```python
from build123d import *

# Parameters (mm, degrees)
SKETCH1_W           = 2500
SKETCH1_H           = 700
SKETCH1_W_2         = 2440
SKETCH1_H_2         = 640
BOSS_EXTRUDE1_DEPTH = 1500
SKETCH2_W           = 2440
SKETCH2_H           = 1440
CUT_EXTRUDE1_DEPTH  = 1500
SKETCH3_W           = 1440
SKETCH3_H           = 640
CUT_EXTRUDE2_DEPTH  = 3595
SKETCH5_W           = 15
SKETCH5_H           = 30
BOSS_EXTRUDE3_DEPTH = 640
BOSS_EXTRUDE4_REACH = 2472
SKETCH7_W           = 30
SKETCH7_H           = 30
SKETCH8_W           = 30
SKETCH8_H           = 30
BOSS_EXTRUDE5_DEPTH = 640


with BuildPart() as part:
    # Sketch1 → Boss-Extrude1 (new body)
    with BuildSketch(Plane.XY):
        with Locations((1250, 350)):
            Rectangle(SKETCH1_W, SKETCH1_H)
        with Locations((1250, 350)):
            Rectangle(SKETCH1_W_2, SKETCH1_H_2, mode=Mode.SUBTRACT)
    extrude(amount=BOSS_EXTRUDE1_DEPTH)

    # Sketch2 → Cut-Extrude1 (cut)
    with BuildSketch(Plane(origin=(0, 700, 0), x_dir=(1, 0, 0), z_dir=(0, 1, 0))):
        with Locations((1250, -750)):
            Rectangle(SKETCH2_W, SKETCH2_H)
    extrude(amount=-CUT_EXTRUDE1_DEPTH, mode=Mode.SUBTRACT)

    # Sketch3 → Cut-Extrude2 (cut)
    with BuildSketch(Plane(origin=(2500, 0, 0), x_dir=(0, 0, -1), z_dir=(1, 0, 0))):
        with Locations((-750, 350)):
            Rectangle(SKETCH3_W, SKETCH3_H)
    extrude(amount=-CUT_EXTRUDE2_DEPTH, mode=Mode.SUBTRACT)

    # Sketch5 → Boss-Extrude3 (add)
    with BuildSketch(Plane(origin=(0, 30, 0), x_dir=(1, 0, 0), z_dir=(0, 1, 0))):
        with Locations((632.5, -15)):
            Rectangle(SKETCH5_W, SKETCH5_H)
        with Locations((647.5, -15)):
            Rectangle(SKETCH5_W, SKETCH5_H)
        with Locations((1242.5, -15)):
            Rectangle(SKETCH5_W, SKETCH5_H)
        with Locations((1257.5, -15)):
            Rectangle(SKETCH5_W, SKETCH5_H)
        Polygon((1860, 0), (1845, 0), (1845, -30), (1860, -30), (1875, -30), (1875, 0), align=None)
        with Locations((1852.5, -1485)):
            Rectangle(SKETCH5_W, SKETCH5_H)
        with Locations((1867.5, -1485)):
            Rectangle(SKETCH5_W, SKETCH5_H)
        with Locations((1242.5, -1485)):
            Rectangle(SKETCH5_W, SKETCH5_H)
        with Locations((1257.5, -1485)):
            Rectangle(SKETCH5_W, SKETCH5_H)
        with Locations((647.5, -1485)):
            Rectangle(SKETCH5_W, SKETCH5_H)
        with Locations((632.5, -1485)):
            Rectangle(SKETCH5_W, SKETCH5_H)
    extrude(amount=BOSS_EXTRUDE3_DEPTH)

    # Sketch7 → Boss-Extrude4 (add, up to next)
    with BuildSketch(Plane(origin=(30, 0, 0), x_dir=(0, 0, -1), z_dir=(1, 0, 0)), mode=Mode.PRIVATE) as boss_extrude4_sk1:
        with Locations((-750, 15)):
            Rectangle(SKETCH7_W, SKETCH7_H)
    boss_extrude4_tool1 = extrude(boss_extrude4_sk1.sketch, amount=BOSS_EXTRUDE4_REACH, mode=Mode.PRIVATE) - part.part
    add(boss_extrude4_tool1.solids().sort_by_distance((30, 15, 750))[0])
    # Sketch7 → Boss-Extrude4 (add, up to next)
    with BuildSketch(Plane(origin=(30, 0, 0), x_dir=(0, 0, -1), z_dir=(1, 0, 0)), mode=Mode.PRIVATE) as boss_extrude4_sk2:
        with Locations((-750, 685)):
            Rectangle(SKETCH7_W, SKETCH7_H)
    boss_extrude4_tool2 = extrude(boss_extrude4_sk2.sketch, amount=BOSS_EXTRUDE4_REACH, mode=Mode.PRIVATE) - part.part
    add(boss_extrude4_tool2.solids().sort_by_distance((30, 685, 750))[0])

    # Sketch8 → Boss-Extrude5 (add)
    with BuildSketch(Plane(origin=(0, 30, 0), x_dir=(1, 0, 0), z_dir=(0, 1, 0))):
        with Locations((2485, -750)):
            Rectangle(SKETCH8_W, SKETCH8_H)
        with Locations((15, -750)):
            Rectangle(SKETCH8_W, SKETCH8_H)
        with Locations((640, -750)):
            Rectangle(SKETCH8_W, SKETCH8_H)
        with Locations((1250, -750)):
            Rectangle(SKETCH8_W, SKETCH8_H)
        with Locations((1860, -750)):
            Rectangle(SKETCH8_W, SKETCH8_H)
    extrude(amount=BOSS_EXTRUDE5_DEPTH)


solid = part.part
```
Geometry: final body of the model. Coordinates: model frame, mm. A direction names the side the tool comes from. Round coordinates to 2 decimals unless told otherwise and drop trailing zeros. Order: outer loops, then holes, each group sorted by start corner. A loop starts at its lowest first (then second) coordinate and runs counter-clockwise, first axis right, second up. Notation, with made-up numbers: (17, 55.25) -> (68, 55.25) arc R31 cw to (68, 86.25) -> close; hole circle Ø8 at (21, 61.5). An arc over 180 degrees is marked (long way). Use CSV: the item, a comma, the result in double quotes. Start each with the question number.
1) Section A-A (z = 680.5). Return the cut outline in (x, y), and give its area (3 significant figures).
2) Section B-B (x = 1768.5). Return the cut outline in (y, z), and give its area (3 significant figures).
3) Set-up query: faces 1 (the face through (0, 322, 746)), 2 (the face through (1244, 352, 1470)). Return all of +Z, -Z, +X, -X, +Y, -Y with unobstructed straight access to the full face (end or side cutting, diameter ignored); none if empty.
4) Draft query along X for faces 3 (the face through (1244, 348, 765)), 4 (the face through (1244, 348, 735)), 5 (the face through (1244, 700, 24)), 6 (the face through (2500, 348, 754)). Return one class per face: +X half, -X half, draft (parallel to the pull), parting line (faces both ways), or undercut.
5) Section C-C (y = 71). State how many separate pieces and enclosed holes the cut face has, and give its area (3 significant figures).
Returned:
1,outline,"(0, 0) -> (30, 0) -> (30, 30) -> (0, 30) -> close; (0, 670) -> (30, 670) -> (30, 700) -> (0, 700) -> close; (2470, 0) -> (2500, 0) -> (2500, 30) -> (2470, 30) -> close; (2470, 670) -> (2500, 670) -> (2500, 700) -> (2470, 700) -> close"
1,area,"3,600 mm²"
2,outline,"(0, 0) -> (30, 0) -> (30, 30) -> (0, 30) -> close; (0, 735) -> (30, 735) -> (30, 765) -> (0, 765) -> close; (0, 1470) -> (30, 1470) -> (30, 1500) -> (0, 1500) -> close; (670, 0) -> (700, 0) -> (700, 30) -> (670, 30) -> close; (670, 735) -> (700, 735) -> (700, 765) -> (670, 765) -> close; (670, 1470) -> (700, 1470) -> (700, 1500) -> (670, 1500) -> close"
2,area,"5,400 mm²"
3,face 1,"+Z, -Z, -X, +Y, -Y"
3,face 2,"+Y, -Y"
4,face 3,"undercut"
4,face 4,"undercut"
4,face 5,"draft"
4,face 6,"+X half"
5,separate pieces,"15"
5,enclosed holes,"0"
5,area,"13,500 mm²"
